Check sheet for the modelled part. Datum: model origin and axes. Units: mm. A direction names the side the tool comes from. Give positions to 0.01 mm unless a question says otherwise; leave off trailing zeros. Order: outer loops, then holes, each group sorted by start corner. A loop starts at its lowest first (then second) coordinate and runs counter-clockwise, first axis right, second up. Notation, with made-up numbers: M -11.5,75.5 L 47.5,75.5 A32 cw 47.5,107.5 Z; hole C 51,60 d3. An arc over 180 degrees is marked long. Answer in a Markdown table with one row per item. Add a question column.
from build123d import *

# Parameters (mm, degrees)
F0_R     = 25.4
F0_R_2   = 1.5875
F0_R_3   = 12.7
F1_DEPTH = 6.35
F2_R     = 19.05
F2_R_2   = 12.7
F3_DEPTH = 25.4
F4_W     = 6.35
F4_H     = 15.4432
F5_DEPTH = 25.401


with BuildPart() as f1:
    # F0 (on Front) → F1 (new body)
    with BuildSketch(Plane.XZ):
        Circle(F0_R)
        with Locations((0, -22.225)):
            Circle(F0_R_2, mode=Mode.SUBTRACT)
        with Locations((-22.225, 0)):
            Circle(F0_R_2, mode=Mode.SUBTRACT)
        Circle(F0_R_3, mode=Mode.SUBTRACT)
        with Locations((22.225, 0)):
            Circle(F0_R_2, mode=Mode.SUBTRACT)
        with Locations((0, 22.225)):
            Circle(F0_R_2, mode=Mode.SUBTRACT)
    extrude(amount=F1_DEPTH)

    # F2 (on Front) → F3 (join)
    with BuildSketch(Plane.XZ):
        Circle(F2_R)
        Circle(F2_R_2, mode=Mode.SUBTRACT)
    extrude(amount=F3_DEPTH)

    # F4 (on Front) → F5 (cut, through all)
    with BuildSketch(Plane.XZ):
        with Locations((0, 7.7216)):
            Rectangle(F4_W, F4_H)
    extrude(amount=F5_DEPTH, mode=Mode.SUBTRACT)


solid = f1.part
Q1. Tool access check on faces 1 (the flat face through (-12, 0, -5)), 2 (the cylindrical face through (-15.12, -15.74, -11.59)), 3 (the flat face through (-3.175, -13, 14)). Record the directions out of +Z, -Z, +X, -X, +Y, -Y that give a thin tool (end or side, any length) a straight path to the whole face; none if there is none.
Q2. Draft check along X on faces 4 (the flat face through (4, -25.4, -12.4)), 5 (the cylindrical face through (-0.51, -12.52, -12.69)), 6 (the cylindrical face through (-5.506, -3.131, -24.796)), 7 (the flat face through (0, -13, 15.443)). Enter one of: pulls with the +X half, pulls with the -X half, needs draft (parallel to the pull), parting line crosses it, or undercut.
Q3. Go/stop test with flat-tipped pins: pin 1 (1.9 mm diameter, centred on x = 1, y = -8, fed in from -Z); pin 2 (4 mm diameter, centred on x = 0, z = -22.225, fed in from -Y); pin 3 (1.6 mm diameter, centred on y = -7.5, z = 13.5, fed in from -X). Record where each tip stops, or that it passes through.
Q4. Cross-section at D-D (z = 10.5). Record the boundary of the cut face in (x, y), and give its area (3 significant figures).
Q5. Cross-section at C-C (y = -8.25). Record the boundary of the cut face in (x, z) (3 decimals), and give its area (3 significant figures).
Q6. Cross-section at A-A (x = 0). Record the boundary of the cut face in (y, z), and give its area (3 significant figures).
Q7. Cross-section at B-B (z = 0). Record the boundary of the cut face in (x, y), and give its area (3 significant figures).
Q8. Thickness scan on probe 1 along Z at (x, y) = (0, -2); probe 2 along Z at (x, y) = (0, -11.75); probe 3 along Y at (x, z) = (-9.5, -23). Record the ranges inside material, lowest first.
Values follow:
| question | item | result |
|---|---|---|
| 1 | face 1 | +Z, -Z, +X, -X, +Y |
| 1 | face 2 | -Y |
| 1 | face 3 | +Y, -Y |
| 2 | face 4 | needs draft |
| 2 | face 5 | undercut |
| 2 | face 6 | parting line crosses it |
| 2 | face 7 | undercut |
| 3 | pin 1 | z = -19.05 |
| 3 | pin 2 | y = -6.35 |
| 3 | pin 3 | x = -14.2 |
| 4 | outline | M -23.13,-6.35 L -15.9,-6.35 L -15.9,-25.4 L -7.14,-25.4 L -7.14,0 L -23.13,0 Z; M 7.14,-25.4 L 15.9,-25.4 L 15.9,-6.35 L 23.13,-6.35 L 23.13,0 L 7.14,0 Z |
| 4 | area | 536 mm² |
| 5 | outline | C 0,0 d38.1; hole M -3.175,12.297 A12.7 ccw long 3.175,12.297 L 3.175,15.443 L -3.175,15.443 Z |
| 5 | area | 615 mm² |
| 6 | outline | M -25.4,-19.05 L -6.35,-19.05 L -6.35,-20.64 L 0,-20.64 L 0,-12.7 L -25.4,-12.7 Z; M -25.4,15.44 L 0,15.44 L 0,20.64 L -6.35,20.64 L -6.35,19.05 L -25.4,19.05 Z; M -6.35,-25.4 L 0,-25.4 L 0,-23.81 L -6.35,-23.81 Z; M -6.35,23.81 L 0,23.81 L 0,25.4 L -6.35,25.4 Z |
| 6 | area | 293 mm² |
| 7 | outline | M -25.4,-6.35 L -23.81,-6.35 L -23.81,0 L -25.4,0 Z; M -20.64,-6.35 L -19.05,-6.35 L -19.05,-25.4 L -12.7,-25.4 L -12.7,0 L -20.64,0 Z; M 12.7,-25.4 L 19.05,-25.4 L 19.05,-6.35 L 20.64,-6.35 L 20.64,0 L 12.7,0 Z; M 23.81,-6.35 L 25.4,-6.35 L 25.4,0 L 23.81,0 Z |
| 7 | area | 363 mm² |
| 8 | probe 1 | -25.4 to -23.81, -20.64 to -12.7, 15.44 to 20.64, 23.81 to 25.4 |
| 8 | probe 2 | -19.05 to -12.7, 15.44 to 19.05 |
| 8 | probe 3 | -6.35 to 0 |
